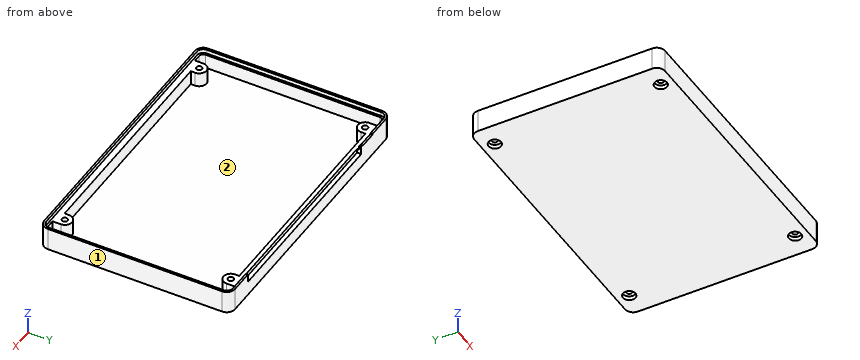
```python
from build123d import *

# Parameters (mm, degrees)
SKETCH1_W           = 137
SKETCH1_H           = 92
BOSS_EXTRUDE1_DEPTH = 2
SKETCH2_W           = 137
SKETCH2_H           = 92
SKETCH2_W_2         = 133
SKETCH2_H_2         = 88
BOSS_EXTRUDE2_DEPTH = 7
SKETCH3_W           = 137
SKETCH3_H           = 92
SKETCH3_W_2         = 135
SKETCH3_H_2         = 90
BOSS_EXTRUDE3_DEPTH = 2
SKETCH4_R           = 1.35
BOSS_EXTRUDE4_DEPTH = 7
SKETCH8_W           = 108
SKETCH8_H           = 1.9
BOSS_EXTRUDE6_DEPTH = 7
FILLET1_R           = 2
FILLET2_R           = 3
FILLET3_R           = 4
SKETCH11_W          = 108
SKETCH11_H          = 1.9
BOSS_EXTRUDE7_DEPTH = 7
SKETCH12_W          = 97
SKETCH12_H          = 4
CUT_EXTRUDE3_DEPTH  = 2
CUT_EXTRUDE4_START  = -10
SKETCH13_R          = 1.35
CUT_EXTRUDE4_DEPTH  = 10
SKETCH14_W          = 8.5
SKETCH14_H          = 0.4
CUT_EXTRUDE5_DEPTH  = 2
SKETCH16_R          = 3
CUT_EXTRUDE12_DEPTH = 2


with BuildPart() as part:
    # Sketch1 → Boss-Extrude1 (new body)
    with BuildSketch(Plane.XY):
        with Locations((68.5, 46)):
            Rectangle(SKETCH1_W, SKETCH1_H)
    extrude(amount=BOSS_EXTRUDE1_DEPTH)

    # Sketch2 → Boss-Extrude2 (add)
    with BuildSketch(Plane.XY.offset(2)):
        with Locations((68.5, 46)):
            Rectangle(SKETCH2_W, SKETCH2_H)
        with Locations((68.5, 46)):
            Rectangle(SKETCH2_W_2, SKETCH2_H_2, mode=Mode.SUBTRACT)
    extrude(amount=BOSS_EXTRUDE2_DEPTH)

    # Sketch3 → Boss-Extrude3 (add)
    with BuildSketch(Plane.XY.offset(9)):
        with Locations((68.5, 46)):
            Rectangle(SKETCH3_W, SKETCH3_H)
        with Locations((68.5, 46)):
            Rectangle(SKETCH3_W_2, SKETCH3_H_2, mode=Mode.SUBTRACT)
    extrude(amount=BOSS_EXTRUDE3_DEPTH)

    # Sketch4 → Boss-Extrude4 (add)
    # profile 1 of 4: a face of its own
    with BuildSketch(Plane.XY.offset(2)):
        with BuildLine():
            Line((7.5, 6), (7.5, 2))
            Line((7.5, 2), (14.5, 2))
            Line((14.5, 2), (14.5, 6))
            ThreePointArc((14.5, 6), (11, 9.5), (7.5, 6))
        make_face()
        with Locations((11, 6)):
            Circle(SKETCH4_R, mode=Mode.SUBTRACT)
    # profile 2 of 4: a face of its own
    with BuildSketch(Plane.XY.offset(2)):
        with BuildLine():
            Line((122.5, 6), (122.5, 2))
            Line((122.5, 2), (129.5, 2))
            Line((129.5, 2), (129.5, 6))
            ThreePointArc((129.5, 6), (126, 9.5), (122.5, 6))
        make_face()
        with Locations((126, 6)):
            Circle(SKETCH4_R, mode=Mode.SUBTRACT)
    # profile 3 of 4: a face of its own
    with BuildSketch(Plane.XY.offset(2)):
        with BuildLine():
            Line((129.5, 86), (129.5, 90))
            Line((129.5, 90), (122.5, 90))
            Line((122.5, 90), (122.5, 86))
            ThreePointArc((122.5, 86), (126, 82.5), (129.5, 86))
        make_face()
        with Locations((126, 86)):
            Circle(SKETCH4_R, mode=Mode.SUBTRACT)
    # profile 4 of 4: a face of its own
    with BuildSketch(Plane.XY.offset(2)):
        with BuildLine():
            Line((14.5, 86), (14.5, 90))
            Line((14.5, 90), (7.5, 90))
            Line((7.5, 90), (7.5, 86))
            ThreePointArc((7.5, 86), (11, 82.5), (14.5, 86))
        make_face()
        with Locations((11, 86)):
            Circle(SKETCH4_R, mode=Mode.SUBTRACT)
    extrude(amount=BOSS_EXTRUDE4_DEPTH)

    # Sketch8 → Boss-Extrude6 (add)
    with BuildSketch(Plane.XY.offset(2)):
        with Locations((68.5, 2.95)):
            Rectangle(SKETCH8_W, SKETCH8_H)
    extrude(amount=BOSS_EXTRUDE6_DEPTH)

    # Fillet1
    fillet1_edges = [part.edges().sort_by_distance(p)[0] for p in [
        (2, 2, 5.5),
        (135, 2, 5.5),
        (135, 90, 5.5),
        (2, 90, 5.5),
    ]]
    fillet(fillet1_edges, radius=FILLET1_R)

    # Fillet2
    fillet2_edges = [part.edges().sort_by_distance(p)[0] for p in [
        (1, 1, 10),
        (136, 1, 10),
        (136, 91, 10),
        (1, 91, 10),
    ]]
    fillet(fillet2_edges, radius=FILLET2_R)

    # Fillet3
    fillet3_edges = [part.edges().sort_by_distance(p)[0] for p in [
        (0, 92, 5.5),
        (137, 92, 5.5),
        (137, 0, 5.5),
        (0, 0, 5.5),
    ]]
    fillet(fillet3_edges, radius=FILLET3_R)

    # Sketch11 → Boss-Extrude7 (add)
    with BuildSketch(Plane.XY.offset(2)):
        with Locations((68.5, 89.05)):
            Rectangle(SKETCH11_W, SKETCH11_H)
    extrude(amount=BOSS_EXTRUDE7_DEPTH)

    # Sketch12 → Cut-Extrude3 (cut)
    with BuildSketch(Plane(origin=(0, 92, 0), x_dir=(1, 0, 0), z_dir=(0, 1, 0))):
        with Locations((73.5, -9)):
            Rectangle(SKETCH12_W, SKETCH12_H)
    extrude(amount=-CUT_EXTRUDE3_DEPTH, mode=Mode.SUBTRACT)

    # Sketch13 → Cut-Extrude4 (cut)
    with BuildSketch(Plane.XY.offset(9).offset(CUT_EXTRUDE4_START)):
        with Locations(Location((11, 86, 0), (0, 0, 180))):
            Circle(SKETCH13_R)
        with Locations(Location((11, 6, 0), (0, 0, 180))):
            Circle(SKETCH13_R)
        with Locations(Location((126, 6, 0), (0, 0, 180))):
            Circle(SKETCH13_R)
        with Locations(Location((126, 86, 0), (0, 0, 180))):
            Circle(SKETCH13_R)
    extrude(amount=CUT_EXTRUDE4_DEPTH, mode=Mode.SUBTRACT)

    # Sketch14 → Cut-Extrude5 (cut)
    with BuildSketch(Plane(origin=(0, 92, 0), x_dir=(1, 0, 0), z_dir=(0, 1, 0))):
        with Locations((19.488221945, -10.8)):
            Rectangle(SKETCH14_W, SKETCH14_H)
    extrude(amount=-CUT_EXTRUDE5_DEPTH, mode=Mode.SUBTRACT)

    # Sketch16 → Cut-Extrude12 (cut)
    with BuildSketch(Plane(origin=(0, 0, 0), x_dir=(-1, 0, 0), z_dir=(0, 0, -1))):
        with Locations((-126, 86)):
            Circle(SKETCH16_R)
        with Locations((-11, 86)):
            Circle(SKETCH16_R)
        with Locations((-11, 6)):
            Circle(SKETCH16_R)
        with Locations((-126, 6)):
            Circle(SKETCH16_R)
    extrude(amount=-CUT_EXTRUDE12_DEPTH, mode=Mode.SUBTRACT)


solid = part.part
```
Model file for the job. Use its own axes, mm. Face numbers are marked on the shaded views. Round coordinates to 2 decimals unless told otherwise and drop trailing zeros. Loops run counter-clockwise (first coordinate to the right, second up) from the corner with the lowest first, then second, coordinate; pieces in that order, holes last. Notation, with made-up numbers: M 14,-36 L 32,-36 A20 ccw 32,-5 Z; hole C -31.5,1.5 d7. An arc over 180 degrees is marked long. Put each result on its own line as item: value. Start each with the question number.
Item 1: Mould opens along Y. For the marked faces 1 and 2 say: released by +Y, released by -Y, zero draft, split by the parting line, or undercut.
Item 2: Cut at B-B (x = 126). List the corners of the cut face in (y, z).
Item 3: Cut at D-D (z = 4). Give the number of separate pieces and of enclosed holes in the cut face, then the cut area to 3 significant figures.
Item 4: Cut at C-C (y = 44.5). List the corners of the cut face in (x, z), then the cut area to 3 significant figures.
Item 5: Cut at A-A (x = 51.5). List the corners of the cut face in (y, z).
Item 6: Drop flat-ended pins along their axis: P1, Ø10, axis at x = 56.5, y = 37, coming from the +Z side; P2, Ø6.5, axis at x = 126.5, y = 5.5, coming from the -Z side; P3, Ø3, axis at x = 11, y = 6, coming from the -Z side; P4, Ø7, axis at x = 11, y = 86, coming from the +Z side. Give the stop position or say it passes through.
Item 7: Drill centre lines: line 1 along Y through (x, z) = (126, 0.7); line 2 along X through (y, z) = (6, 7.75); line 3 along X through (y, z) = (55, 9.25). Where is each one in solid material? Low to high.
Answer block:
1. face 1: zero draft
1. face 2: undercut
2. outline: M 0,0 L 3,0 L 3,2 L 4.65,2 L 4.65,9 L 1,9 L 1,11 L 0,11 Z; M 7.35,2 L 9,2 L 9,0 L 83,0 L 83,2 L 84.65,2 L 84.65,9 L 82.5,9 L 82.5,2 L 9.5,2 L 9.5,9 L 7.35,9 Z; M 87.35,2 L 89,2 L 89,0 L 92,0 L 92,11 L 91,11 L 91,9 L 87.35,9 Z
3. separate pieces: 1
3. enclosed holes: 5
3. area: 1,470 mm2
4. outline: M 0,0 L 137,0 L 137,11 L 136,11 L 136,9 L 135,9 L 135,2 L 2,2 L 2,9 L 1,9 L 1,11 L 0,11 Z
4. area: 306 mm2
5. outline: M 0,0 L 92,0 L 92,7 L 90,7 L 90,9 L 88.1,9 L 88.1,2 L 3.9,2 L 3.9,9 L 1,9 L 1,11 L 0,11 Z
6. P1: z = 2
6. P2: z = 0
6. P3: z = 2
6. P4: z = 9
7. line 1: 0 to 3, 9 to 83, 89 to 92
7. line 2: 0 to 2, 7.5 to 9.65, 12.35 to 14.5, 122.5 to 124.65, 127.35 to 129.5, 135 to 137
7. line 3: 0 to 1, 136 to 137
